Check sheet for the modelled part. Datum: model origin and axes. Units: mm. Face numbers are marked on the shaded views. A direction names the side the tool comes from. Give positions to 0.01 mm unless a question says otherwise; leave off trailing zeros. Order: outer loops, then holes, each group sorted by start corner. A loop starts at its lowest first (then second) coordinate and runs counter-clockwise, first axis right, second up. Notation, with made-up numbers: M 28.25,8.25 L 68.25,8.25 A24 ccw 68.25,44.25 Z; hole C 41.25,22 d4. An arc over 180 degrees is marked long. One line per question, with ' | ' between items. Start each with the question number.
```python
from build123d import *

# Parameters (mm, degrees)
F1_DEPTH = 25.4
F3_DEPTH = 25.4
F4_W     = 12.7
F4_H     = 6.3569043029
F5_DEPTH = 38.1


with BuildPart() as f1:
    # F0 (on Front) → F1 (new body)
    with BuildSketch(Plane.XZ):
        Polygon((-22.4366684005, 65.2284603763), (-60.5366684005, 65.2284603763), (-60.5366684005, 27.1284603763), (-22.4366684005, 26.9258023975), align=None)
    extrude(amount=F1_DEPTH)

    # F2 (on face) → F3 (cut)
    with BuildSketch(Plane.XZ.offset(25.4)):
        Polygon((-47.3802936689, 33.2767914322), (-47.4133685962, 27.0586561397), (-35.7620950777, 26.9966817686), (-35.7620950777, 33.2149929902), align=None)
    extrude(amount=-F3_DEPTH, mode=Mode.SUBTRACT)

    # F4 (on face) → F5 (cut)
    with BuildSketch(Plane.YZ.offset(-22.4366684005)):
        with Locations((-12.7, 62.0500082249)):
            Rectangle(F4_W, F4_H)
    extrude(amount=-F5_DEPTH, mode=Mode.SUBTRACT)


solid = f1.part
```
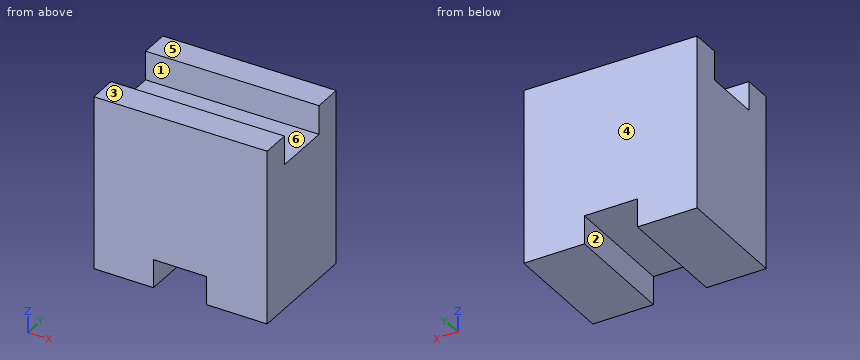
Item 1: Set-up check for the marked faces 1, 2 and 3: record each of +Z, -Z, +X, -X, +Y, -Y from which the full face is reachable in a straight line by a thin tool's end or side.
Item 2: Section check B-B, the plane z = 31.5. Record the cut outline in (x, y), then the cut area to 3 significant figures.
Item 3: Draft check along Y on the marked faces 4, 5 and 6. Enter one of: released by +Y, released by -Y, zero draft, split by the parting line, or undercut.
Item 4: Section check C-C, the plane x = -50. Record the cut outline in (y, z).
Item 5: Section check A-A, the plane y = -11.75. Record the cut outline in (x, z) (3 decimals), then the cut area to 3 significant figures.
Item 6: Go/stop test with flat-tipped pins: P1, Ø4, axis at x = -34, y = -7, coming from the -Z side; P2, Ø4, axis at x = -30, y = -9.5, coming from the +Z side; P3, Ø5, axis at x = -41.5, y = -13.5, coming from the -Z side. Record where each tip stops, or that it passes through.
Item 7: Scan lines: probe 1 along X at (y, z) = (-8.25, 33); probe 2 along Z at (x, y) = (-31, -22.5); probe 3 along Z at (x, y) = (-51.5, -12.25). Record each from-to range of solid material in increasing order. Write a range as [from, to].
Reported:
1) face 1: +Z, +X, -X | face 2: -Z, +Y, -Y | face 3: +Z, +X, -X, +Y, -Y
2) outline: M -60.54,-25.4 L -47.39,-25.4 L -47.39,0 L -60.54,0 Z; M -35.76,-25.4 L -22.44,-25.4 L -22.44,0 L -35.76,0 Z | area: 672 mm^2
3) face 4: released by +Y | face 5: zero draft | face 6: undercut
4) outline: M -25.4,27.07 L 0,27.07 L 0,65.23 L -6.35,65.23 L -6.35,58.87 L -19.05,58.87 L -19.05,65.23 L -25.4,65.23 Z
5) outline: M -60.537,27.128 L -47.413,27.059 L -47.38,33.277 L -35.762,33.215 L -35.762,26.997 L -22.437,26.926 L -22.437,58.872 L -60.537,58.872 Z | area: 1,140 mm^2
6) P1: stops at z = 26.98 | P2: stops at z = 58.87 | P3: stops at z = 33.23
7) probe 1: x = [-60.54, -47.38], [-35.76, -22.44] | probe 2: z = [26.97, 65.23] | probe 3: z = [27.08, 58.87]
